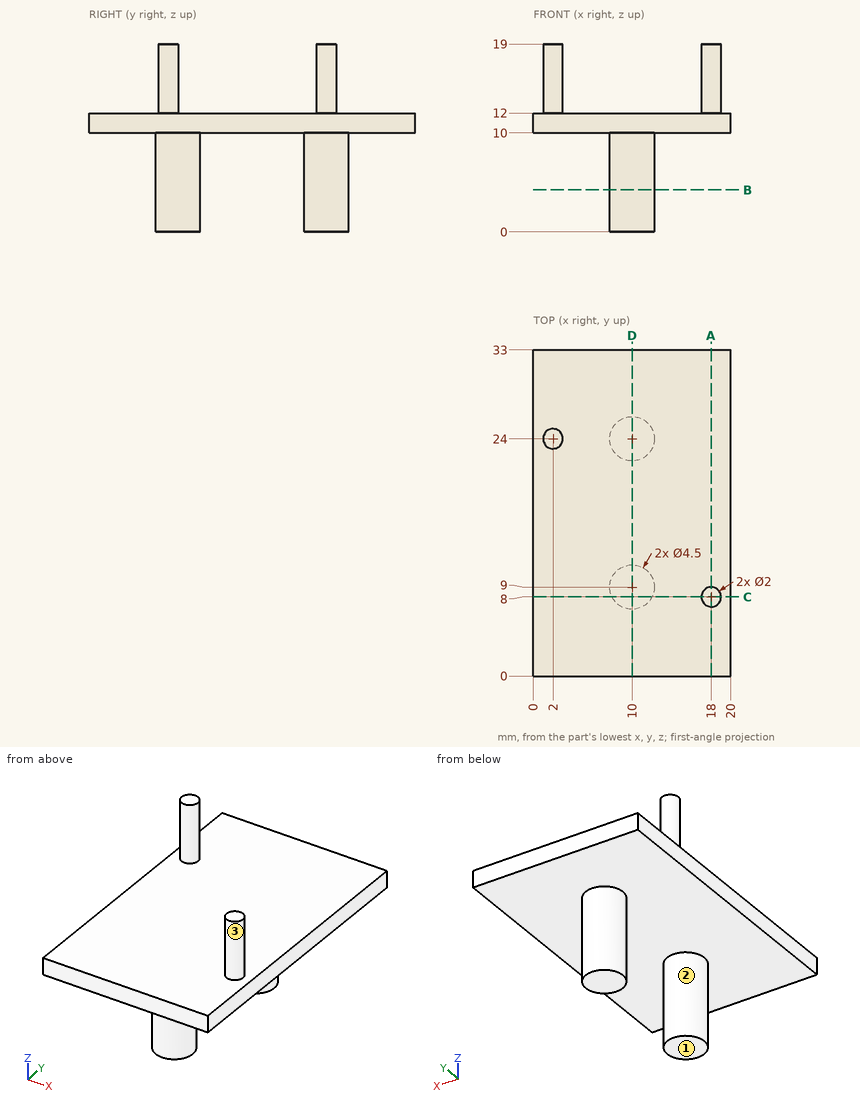
Study the drawing (mm; zero at the part's minimum x, y, z) and answer. A direction names the side the tool comes from. Give positions to 0.01 mm unless a question says otherwise; leave off trailing zeros. Write each loop counter-clockwise with the first axis right and the second up, starting at its lowest first coordinate (ties: lowest second). Pieces come first, ordered by that corner, then holes. Notation, with made-up numbers: (54.5, 0.25) - (103.5, 0.25) arc R14 ccw to (103.5, 19.25) - close; hole circle Ø7 at (-19, 77.5). An arc over 180 degrees is marked (long way). Write item = value, one per line. Start each with the question number.
Item 1: Each of these flat-tipped pins is pushed along its axis until it touches: P1, Ø8, axis at y = 24.5, z = 15.5, coming from the -X side; P2, Ø1.5, axis at x = 9, y = 26.5, coming from the +Z side; P3, Ø3, axis at y = 10.5, z = 5.5, coming from the +X side; P4, Ø3, axis at x = 9, y = 29.5, coming from the -Z side. Where does it stop, or does it pass through?
Item 2: Find the intervals of material crossed by probe 1 along Z at (x, y) = (14.5, 17); probe 2 along Z at (x, y) = (2.5, 24); probe 3 along Y at (x, z) = (11.5, 7), in increasing order. Write a range as [from, to].
Item 3: Find section B-B (z = 4.25). Give the vertices of the cut face in (x, y).
Item 4: Find section C-C (y = 8). Give the vertices of the cut face in (x, z).
Item 5: Find section A-A (x = 18). Give the vertices of the cut face in (y, z).
Item 6: A tool of negligible diameter and unlimited length cuts with its end or side. For the marked faces 1, 2 and 3, from which of +Z, -Z, +X, -X, +Y, -Y can it reach the whole face along a straight path? Write none if from no direction.
Item 7: Find section D-D (x = 10). Give the vertices of the cut face in (y, z).
Response:
q1.P1 = 0
q1.P2 = 12
q1.P3 = 12.25
q1.P4 = 10
q2.probe_1 = [10, 12]
q2.probe_2 = [10, 19]
q2.probe_3 = [7.32, 10.68], [22.32, 25.68]
q3.outline = circle Ø4.5 at (10, 9); circle Ø4.5 at (10, 24)
q4.outline = (0, 10) - (7.98, 10) - (7.98, 0) - (12.02, 0) - (12.02, 10) - (20, 10) - (20, 12) - (19, 12) - (19, 19) - (17, 19) - (17, 12) - (0, 12) - close
q5.outline = (0, 10) - (33, 10) - (33, 12) - (9, 12) - (9, 19) - (7, 19) - (7, 12) - (0, 12) - close
q6.face_1 = -Z, +X, -X, +Y, -Y
q6.face_2 = -Z
q6.face_3 = +Z
q7.outline = (0, 10) - (6.75, 10) - (6.75, 0) - (11.25, 0) - (11.25, 10) - (21.75, 10) - (21.75, 0) - (26.25, 0) - (26.25, 10) - (33, 10) - (33, 12) - (0, 12) - close
